Design review of the part built by this model. Coordinates are the model's own, in mm. A direction names the side the tool comes from. Round coordinates to 2 decimals unless told otherwise and drop trailing zeros. Order: outer loops, then holes, each group sorted by start corner. A loop starts at its lowest first (then second) coordinate and runs counter-clockwise, first axis right, second up.
from build123d import *

# Parameters (mm, degrees)
F0_W      = 76.2
F0_H      = 76.2
F1_DEPTH  = 76.2
F2_R      = 2.54
F3_R      = 5.08
F4_DEPTH  = 10.16
F5_R      = 6.35
F6_DEPTH  = 12.7
F6_FACE_R = 6.35
F7_DEPTH  = 2540
F8_R      = 6.35
F9_DEPTH  = 12.7
F10_R     = 6.35
F11_DEPTH = 10.16
F12_R     = 6.35
F13_DEPTH = 10.16
F14_R     = 6.35
F15_DEPTH = 10.16


with BuildPart() as f1:
    # F0 (on Front) → F1 (new body)
    with BuildSketch(Plane.XZ):
        Rectangle(F0_W, F0_H)
    extrude(amount=F1_DEPTH)

    # F2
    f2_edges = [f1.edges().sort_by_distance(p)[0] for p in [
        (0, 0, 38.1),
        (-38.1, -38.1, 38.1),
        (-38.1, 0, 0),
        (-38.1, -76.2, 0),
        (0, -76.2, 38.1),
        (0, -76.2, -38.1),
        (38.1, -76.2, 0),
        (-38.1, -38.1, -38.1),
        (38.1, -38.1, -38.1),
        (0, 0, -38.1),
        (38.1, 0, 0),
        (38.1, -38.1, 38.1),
    ]]
    fillet(f2_edges, radius=F2_R)

    # F3 (on face) → F4 (cut)
    with BuildSketch(Plane.XY.offset(38.1)):
        with Locations((0, -39.432134)):
            Circle(F3_R)
    extrude(amount=-F4_DEPTH, mode=Mode.SUBTRACT)

    # F5 (on face) → F6 (cut)
    with BuildSketch(Plane.XZ.offset(76.2)):
        with Locations((-18.525468, -19.626983)):
            Circle(F5_R)
        with Locations((17.524092, 17.22368)):
            Circle(F5_R)
        Circle(F5_R)
    extrude(amount=-F6_DEPTH, mode=Mode.SUBTRACT)

    # F6_face (on face) → F7 (cut)
    with BuildSketch(Plane.XZ.offset(63.5)):
        Circle(F6_FACE_R)
    extrude(amount=-F7_DEPTH, mode=Mode.SUBTRACT)

    # F8 (on face) → F9 (cut)
    with BuildSketch(Plane(origin=(0, 0, 0), x_dir=(-1, 0, 0), z_dir=(0, 1, 0))):
        with Locations((-18.926021, 17.423956)):
            Circle(F8_R)
        with Locations((18.307427, 17.491662)):
            Circle(F8_R)
        with Locations((-18.594825, -16.969131)):
            Circle(F8_R)
        with Locations((19.088846, -16.791513)):
            Circle(F8_R)
    extrude(amount=-F9_DEPTH, mode=Mode.SUBTRACT)

    # F10 (on face) → F11 (cut)
    with BuildSketch(Plane(origin=(0, 0, -38.1), x_dir=(1, 0, 0), z_dir=(0, 0, -1))):
        with Locations((-19.3006, 59.993013)):
            Circle(F10_R)
        with Locations((-18.899389, 41.696207)):
            Circle(F10_R)
        with Locations((16.964177, 60.541245)):
            Circle(F10_R)
        with Locations((17.018, 42.472795)):
            Circle(F10_R)
        with Locations((17.969948, 23.708652)):
            Circle(F10_R)
        with Locations((-18.581695, 22.98594)):
            Circle(F10_R)
    extrude(amount=-F11_DEPTH, mode=Mode.SUBTRACT)

    # F12 (on face) → F13 (cut)
    with BuildSketch(Plane.YZ.offset(38.1)):
        with Locations((-22.802937, 17.738998)):
            Circle(F12_R)
        with Locations((-54.048792, -18.630479)):
            Circle(F12_R)
    extrude(amount=-F13_DEPTH, mode=Mode.SUBTRACT)

    # F14 (on face) → F15 (cut)
    with BuildSketch(Plane(origin=(-38.1, 0, 0), x_dir=(0, -1, 0), z_dir=(-1, 0, 0))):
        with Locations((21.129049, 20.828636)):
            Circle(F14_R)
        with Locations((50.461128, 20.828636)):
            Circle(F14_R)
        with Locations((21.129049, -15.14654)):
            Circle(F14_R)
        with Locations((50.461128, -15.14654)):
            Circle(F14_R)
        with Locations((35.348602, 0)):
            Circle(F14_R)
    extrude(amount=-F15_DEPTH, mode=Mode.SUBTRACT)


solid = f1.part
1) For faces 5 (the face through (-19, -12.7, -17)), 6 (the face through (18, -24, -27.94)), 7 (the face through (-27.94, -35, 0)), 8 (the face through (-12.47, -69.94, -17.72)), list the 3-axis set-ups (+Z, -Z, +X, -X, +Y, -Y) from which the entire face can be reached by the end or side of a thin tool; tool diameter is ignored.
Results:
face 5: +Y
face 6: -Z
face 7: -X
face 8: -Y
2) Take a section at A-A on x = 0. Give the boundary of the cut face in (y, z).
Results:
outline: (-76.2, -35.56) arc R2.54 ccw to (-73.66, -38.1) - (-2.54, -38.1) arc R2.54 ccw to (0, -35.56) - (0, -6.35) - (-76.2, -6.35) - close; (-76.2, 6.35) - (0, 6.35) - (0, 35.56) arc R2.54 ccw to (-2.54, 38.1) - (-34.35, 38.1) - (-34.35, 27.94) - (-44.51, 27.94) - (-44.51, 38.1) - (-73.66, 38.1) arc R2.54 ccw to (-76.2, 35.56) - close
3) Clearance check with flat-ended pins moving along their axes: P1, Ø10, axis at x = -21, y = -59, coming from the -Z side; P2, Ø1, axis at x = 14, z = -16.5, coming from the +Y side; P3, Ø4, axis at x = 17.5, y = -43.5, coming from the -Z side; P4, Ø6.5, axis at y = -21, z = -16.5, coming from the -X side. State where each tip first meets the part, or that it passes through.
Results:
P1: stops at z = -38.1
P2: stops at y = -12.7
P3: stops at z = -27.94
P4: stops at x = -27.94
4) To check wall thickness, follow line 1 along Z through (x, y) = (0, -59.5); line 2 along X through (y, z) = (-43, -28.5); line 3 along Z through (x, y) = (-23.5, -10.5). State the ranges of each line that lie inside material, in increasing order.
Results:
line 1: z = -38.1 to -6.35, 6.35 to 38.1
line 2: x = -38.1 to -25.11, -12.68 to 10.69, 23.35 to 38.1
line 3: z = -38.1 to -21.36, -12.22 to 13.84, 21.15 to 38.1
5) Take a section at C-C on x = 32. Give the boundary of the cut face in (y, z).
Results:
outline: (-76.2, -35.56) arc R2.54 ccw to (-73.66, -38.1) - (-2.54, -38.1) arc R2.54 ccw to (0, -35.56) - (0, 35.56) arc R2.54 ccw to (-2.54, 38.1) - (-73.66, 38.1) arc R2.54 ccw to (-76.2, 35.56) - close; hole circle Ø12.7 at (-54.05, -18.63); hole circle Ø12.7 at (-22.8, 17.74)
6) Take a section at B-B on z = 0. Give the boundary of the cut face in (x, y).
Results:
outline: (-38.1, -73.66) arc R2.54 ccw to (-35.56, -76.2) - (-6.35, -76.2) - (-6.35, 0) - (-35.56, 0) arc R2.54 ccw to (-38.1, -2.54) - (-38.1, -29) - (-27.94, -29) - (-27.94, -41.7) - (-38.1, -41.7) - close; (6.35, -76.2) - (35.56, -76.2) arc R2.54 ccw to (38.1, -73.66) - (38.1, -2.54) arc R2.54 ccw to (35.56, 0) - (6.35, 0) - close
7) Take a section at D-D on y = -68. Give the boundary of the cut face in (x, z).
Results:
outline: (-38.1, -35.56) arc R2.54 ccw to (-35.56, -38.1) - (35.56, -38.1) arc R2.54 ccw to (38.1, -35.56) - (38.1, 35.56) arc R2.54 ccw to (35.56, 38.1) - (-35.56, 38.1) arc R2.54 ccw to (-38.1, 35.56) - close; hole circle Ø12.7 at (-18.53, -19.63); hole circle Ø12.7 at (0, 0); hole circle Ø12.7 at (17.52, 17.22)
8) The part is to be moulded in two halves that separate along Z. For faces 1 (the face through (-27.94, -21, -15)), 2 (the face through (37.376, -75.436, 0.498)), 3 (the face through (17, -43, -27.94)), 4 (the face through (37.376, -38.598, 37.336)), say which applies: released by +Z, released by -Z, zero draft, split by the parting line, or undercut.
Results:
face 1: undercut
face 2: zero draft
face 3: released by -Z
face 4: released by +Z
